Answer from the drawing. Dimensions are ordinates in mm from the lowest x, y and z of the part. A direction names the side the tool comes from. Round coordinates to 2 decimals unless told otherwise and drop trailing zeros. Write each loop counter-clockwise with the first axis right and the second up, starting at its lowest first coordinate (ties: lowest second). Pieces come first, ordered by that corner, then holes. Notation, with made-up numbers: (84.5, -0.5) -> (136.5, -0.5) arc R17 cw to (136.5, 16.5) -> close; hole circle Ø6 at (-13, 77). An arc over 180 degrees is marked (long way). Answer as a JSON object with one key per item and string values. Group by question number.
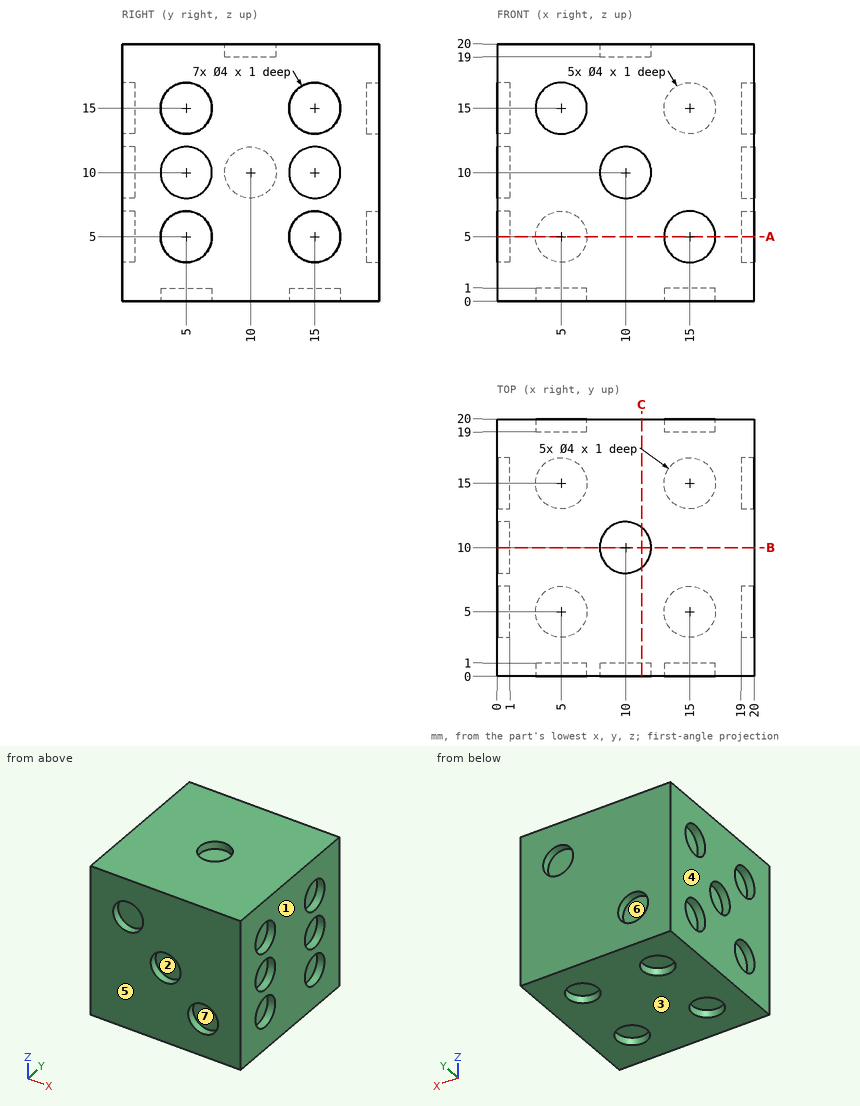
1) Each of these flat-tipped pins is pushed along its axis until it touches: P1, Ø1.2, axis at y = 5.5, z = 14, coming from the -X side; P2, Ø2, axis at x = 4.5, y = 5.5, coming from the -Z side; P3, Ø2, axis at y = 5.5, z = 15, coming from the +X side. Where does it stop, or does it pass through?
2) Straight lines are drawn through the part: L1, parallel to Y at x = 15, z = 0.35; L2, parallel to Z at x = 19.8, y = 15. For each, find the intervals that lie inside material, in ascending order.
3) A cutting plane is placed at C-C on x = 11.25. Determine the outline of the cut face in (y, z), plus the area to 3 significant figures.
4) A cutting plane is placed at A-A on z = 5. Determine the outline of the cut face in (x, y).
5) A tool of negligible diameter and unlimited length cuts with its end or side. For the marked faces 5, 6 and 7, from which of +Z, -Z, +X, -X, +Y, -Y can it reach the whole face along a straight path? Write none if from no direction.
6) For a pull along X with two mould halves and no side action, classify the marked faces 1, 2, 3 and 4 as released by +X, released by -X, zero draft, split by the parting line, or undercut.
7) A cutting plane is placed at B-B on y = 10. Determine the outline of the cut face in (x, z), plus the area to 3 significant figures.
Established:
{
 "1": {"P1": "stops at x = 1", "P2": "stops at z = 1", "P3": "stops at x = 19"},
 "2": {"L1": "y = 0 to 3, 7 to 13, 17 to 20", "L2": "z = 0 to 3, 7 to 8, 12 to 13, 17 to 20"},
 "3": {"outline": "(0, 0) -> (20, 0) -> (20, 20) -> (11.56, 20) -> (11.56, 19) -> (8.44, 19) -> (8.44, 20) -> (0, 20) -> (0, 11.56) -> (1, 11.56) -> (1, 8.44) -> (0, 8.44) -> close", "area": "394 mm²"},
 "4": {"outline": "(0, 0) -> (13, 0) -> (13, 1) -> (17, 1) -> (17, 0) -> (20, 0) -> (20, 3) -> (19, 3) -> (19, 7) -> (20, 7) -> (20, 13) -> (19, 13) -> (19, 17) -> (20, 17) -> (20, 20) -> (7, 20) -> (7, 19) -> (3, 19) -> (3, 20) -> (0, 20) -> (0, 17) -> (1, 17) -> (1, 13) -> (0, 13) -> (0, 7) -> (1, 7) -> (1, 3) -> (0, 3) -> close"},
 "5": {"face 5": "+Z, -Z, +X, -X, -Y", "face 6": "+Y", "face 7": "-Y"},
 "6": {"face 1": "released by +X", "face 2": "undercut", "face 3": "zero draft", "face 4": "released by -X"},
 "7": {"outline": "(0, 0) -> (20, 0) -> (20, 20) -> (12, 20) -> (12, 19) -> (8, 19) -> (8, 20) -> (0, 20) -> (0, 12) -> (1, 12) -> (1, 8) -> (0, 8) -> close", "area": "392 mm²"}
}
